Geometry check sheet. Reference: the model listing, model coordinates, mm. Face numbers are marked on the shaded views. A direction names the side the tool comes from. Coordinates: 2 decimals unless noted, no trailing zeros. Write each loop counter-clockwise with the first axis right and the second up, starting at its lowest first coordinate (ties: lowest second). Pieces come first, ordered by that corner, then holes. Notation, with made-up numbers: M -3.5,-0.5 L 14.5,-0.5 A20 ccw 14.5,29.5 Z; hole C 42,-1 d10. An arc over 180 degrees is marked long. Answer as a JSON object with one key per item and string values. Group by question number.
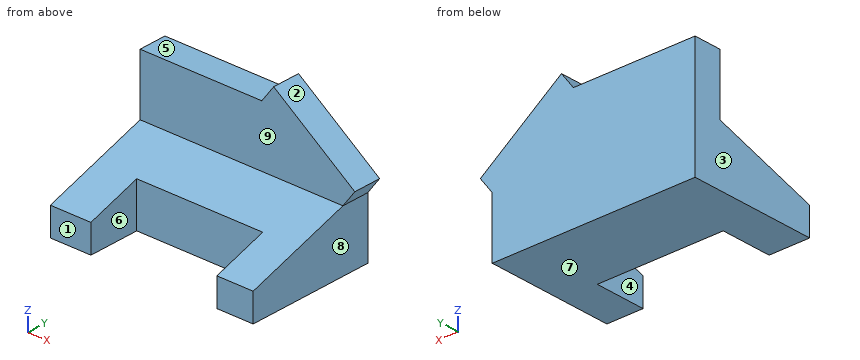
```python
from build123d import *

# Parameters (mm, degrees)
F1_DEPTH = 95
F3_DEPTH = 13.001
F4_W     = 59
F4_H     = 24
F5_DEPTH = 56.001
F6_DEPTH = 9.4


# Not quite as in the source:
# - a feature names something its author has since deleted; it is built from what else it names


with BuildPart() as f1:
    # F0 (on Right) → F1 (new body)
    with BuildSketch(Plane.YZ):
        Polygon((-60, 13), (-60, 0), (0, 0), (0, 56), (-13, 56), (-13, 28), align=None)
    extrude(amount=F1_DEPTH)

    # F2 (on face) → F3 (cut, through all)
    with BuildSketch(Plane.XZ.offset(13)):
        Polygon((95, 56), (57, 56), (95, 28), align=None)
    extrude(amount=-F3_DEPTH, mode=Mode.SUBTRACT)

    # F4 (on face) → F5 (cut, through all)
    with BuildSketch(Plane(origin=(0, 0, 0), x_dir=(1, 0, 0), z_dir=(0, 0, -1))):
        with Locations((48.5, 48)):
            Rectangle(F4_W, F4_H)
    extrude(amount=-F5_DEPTH, mode=Mode.SUBTRACT)

    # F6 (add): a face of the model
    f6_faces = [f1.faces().sort_by_distance(p)[0] for p in [
        (76, -6.5, 42),
    ]]
    extrude(f6_faces, amount=F6_DEPTH)


solid = f1.part
```
1) Section check A-A (x = 17). Record the cut outline in (y, z).
2) Section check D-D (y = -8). Record the cut outline in (x, z), then the cut area to 3 significant figures.
3) Section check B-B (y = -47). Record the cut outline in (x, z), then the cut area to 3 significant figures.
4) Material ranges on probe 1 along X at (y, z) = (-48.5, 16.5); probe 2 along Y at (x, z) = (56, 40.5); probe 3 along Y at (x, z) = (73, 20.5), recorded low to high. Write a range as [from, to].
5) Draft check along X on the marked faces 1, 2, 3 and 4. Enter one of: +X half, -X half, draft (parallel to the pull), parting line (faces both ways), or undercut.
6) Section check C-C (z = 19). Record the cut outline in (x, y).
7) Set-up check for the marked faces 5, 6, 7, 8 and 9: record each of +Z, -Z, +X, -X, +Y, -Y from which the full face is reachable in a straight line by a thin tool's end or side.
8) Go/stop test with flat-tipped pins: pin 1 Ø8.5 at (y, z) = (-25, 14) entering from +X; pin 2 Ø2 at (x, z) = (67.5, 50) entering from -Y; pin 3 Ø10.5 at (x, y) = (27.5, -9.5) entering from +Z. Record where each tip stops, or that it passes through.
Entries:
{
 "1": {"outline": "M -60,0 L 0,0 L 0,56 L -13,56 L -13,28 L -60,13 Z"},
 "2": {"outline": "M 0,0 L 95,0 L 95,28 L 100.58,35.57 L 62.58,63.57 L 57,56 L 0,56 Z", "area": "5,230 mm^2"},
 "3": {"outline": "M 0,0 L 19,0 L 19,17.15 L 0,17.15 Z; M 78,0 L 95,0 L 95,17.15 L 78,17.15 Z", "area": "617 mm^2"},
 "4": {"probe 1": "[0, 19], [78, 95]", "probe 2": "[-13, 0]", "probe 3": "[-36, 0]"},
 "5": {"face 1": "draft", "face 2": "+X half", "face 3": "-X half", "face 4": "undercut"},
 "6": {"outline": "M 0,-41.2 L 19,-41.2 L 19,-36 L 78,-36 L 78,-41.2 L 95,-41.2 L 95,0 L 0,0 Z"},
 "7": {"face 5": "+Z, -X, +Y, -Y", "face 6": "+Z, -Z, -Y", "face 7": "-Z, +X, -X, +Y, -Y", "face 8": "-Z, +X, +Y, -Y", "face 9": "+Z, +X, -X, -Y"},
 "8": {"pin 1": "x = 95", "pin 2": "y = -13", "pin 3": "z = 56"}
}
